from build123d import *

# Parameters (mm, degrees)
EXTRUDE_1_DEPTH          = 20
SKETCH_3_W               = 35
SKETCH_3_H               = 20
EXTRUDE_2_DEPTH          = 5
SKETCH_4_W               = 15
SKETCH_4_H               = 10
EXTRUDE_3_DEPTH          = 5
FILLET_1_R               = 10
CUT_EXTRUDE_1_DEPTH      = 46
CUT_EXTRUDE_1_DEPTH_BACK = 46
SKETCH_5_W               = 10
SKETCH_5_H               = 20
SKETCH_6_R               = 2.5
CUT_EXTRUDE_2_DEPTH      = 5


with BuildPart() as part:
    # 草圖1 → 填料-伸長1 (new body)
    with BuildSketch(Plane(origin=(0, 0, 0), x_dir=(0, 0, -1), z_dir=(1, 0, 0))):
        Polygon((-10, 20), (-20, 5), (-20, 0), (0, 0), (0, 20), align=None)
    extrude(amount=EXTRUDE_1_DEPTH)

    # 草圖3 → 填料-伸長2 (add)
    with BuildSketch(Plane.XZ):
        with Locations((17.5, 10)):
            Rectangle(SKETCH_3_W, SKETCH_3_H)
    extrude(amount=EXTRUDE_2_DEPTH)

    # 草圖4 → 填料-伸長3 (add)
    with BuildSketch(Plane(origin=(0, 0, 0), x_dir=(-1, 0, 0), z_dir=(0, 0, -1))):
        with Locations((-27.5, 5)):
            Rectangle(SKETCH_4_W, SKETCH_4_H)
    extrude(amount=-EXTRUDE_3_DEPTH)

    # 圓角1
    fillet_1_edges = [part.edges().sort_by_distance(p)[0] for p in [
        (35, 10, 2.5),
    ]]
    fillet(fillet_1_edges, radius=FILLET_1_R)

    # 草圖5 → 除料-伸長1 (cut, two sides: drawn at the far end of the back side and taken through both)
    with BuildSketch(Plane.XY.offset(-CUT_EXTRUDE_1_DEPTH_BACK)):
        with Locations((10, 20)):
            Rectangle(SKETCH_5_W, SKETCH_5_H)
    extrude(amount=CUT_EXTRUDE_1_DEPTH + CUT_EXTRUDE_1_DEPTH_BACK, mode=Mode.SUBTRACT)

    # 草圖6 → 除料-伸長2 (cut)
    with BuildSketch(Plane(origin=(0, 0, 0), x_dir=(1, 0, 0), z_dir=(0, 1, 0))):
        with Locations(Location((27.5, -12.5, 0), (0, 0, 270))):
            Circle(SKETCH_6_R)
    extrude(amount=-CUT_EXTRUDE_2_DEPTH, mode=Mode.SUBTRACT)


solid = part.part
Model file for the job. Use its own axes, mm. A direction names the side the tool comes from. Coordinates: 2 decimals unless noted, no trailing zeros. Write each loop counter-clockwise with the first axis right and the second up, starting at its lowest first coordinate (ties: lowest second). Pieces come first, ordered by that corner, then holes. Notation, with made-up numbers: (-21, 25) -> (15, 25) arc R16 cw to (15, 36) -> close; hole circle Ø1 at (51.25, -6). An arc over 180 degrees is marked (long way). One line per item, written item: value. Start each with the question number.
1) Slice it at D-D on z = 6.75. Write the cut outline in (x, y), then the cut area to 3 significant figures.
2) Pull direction X, two halves, no side cores. Call faces 4 (the face through (18, 5, 0)), 5 (the face through (35, -3, 10)), 6 (the face through (10, 10, 8)): +X half, -X half, draft (parallel to the pull), parting line (faces both ways), or undercut.
3) Slice it at A-A on z = 12.5. Write the cut outline in (x, y), then the cut area to 4 significant figures.
4) Slice it at B-B on y = 15. Write the cut outline in (x, z), then the cut area to 3 significant figures.
5) Flat gauge pins, fed straight in: pin 1 Ø3 at (x, z) = (17.5, 15) entering from +Y; pin 2 Ø5 at (x, z) = (12, 5) entering from +Y; pin 3 Ø1 at (y, z) = (16, 12.5) entering from +X. Where does each tip first touch, or does it go through?
6) Which spindle directions (+Z, -Z, +X, -X, +Y, -Y) get a long thin tool onto all of the face, cutting with end or side? Do faces 1 (the face through (15, 15, 6)), 2 (the face through (27, 0, 16)), 3 (the face through (23, 10, 2)). Say none if no direction does.
7) Slice it at C-C on x = 17. Write the cut outline in (y, z), then the cut area to 3 significant figures.
8) Probe probe 1 along X at (y, z) = (-2.8, 12.5); probe 2 along X at (y, z) = (11.5, 5.75); probe 3 along Y at (x, z) = (10, 13.75). List the from-to ranges inside material, lowest first.
Answers follow:
1. outline: (0, -5) -> (35, -5) -> (35, 0) -> (20, 0) -> (20, 20) -> (15, 20) -> (15, 10) -> (5, 10) -> (5, 20) -> (0, 20) -> close
1. area: 475 mm2
2. face 4: draft
2. face 5: +X half
2. face 6: undercut
3. outline: (0, -5) -> (25, -5) -> (25, 0) -> (20, 0) -> (20, 16.25) -> (15, 16.25) -> (15, 10) -> (5, 10) -> (5, 16.25) -> (0, 16.25) -> close; (30, -5) -> (35, -5) -> (35, 0) -> (30, 0) -> close
3. area: 412.5 mm2
4. outline: (0, 0) -> (5, 0) -> (5, 13.33) -> (0, 13.33) -> close; (15, 0) -> (20, 0) -> (20, 13.33) -> (15, 13.33) -> close
4. area: 133 mm2
5. pin 1: y = 14.75
5. pin 2: y = 10
5. pin 3: x = 20
6. face 1: +Z, -Z, +Y
6. face 2: +Z, +X, +Y
6. face 3: +Z, -Z, +X, +Y
7. outline: (-5, 0) -> (20, 0) -> (20, 10) -> (5, 20) -> (-5, 20) -> close
7. area: 425 mm2
8. probe 1: 0 to 25, 30 to 35
8. probe 2: 0 to 5, 15 to 20
8. probe 3: -5 to 10
